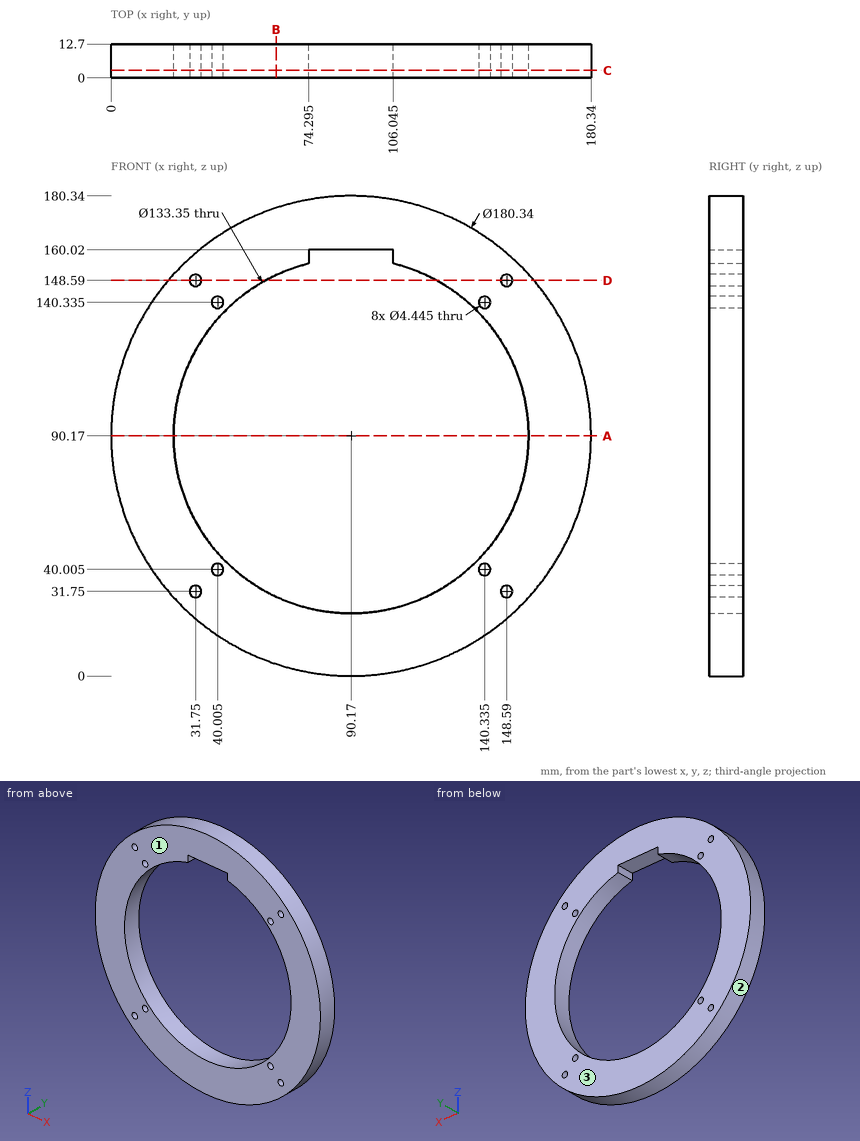
Study the drawing (mm; zero at the part's minimum x, y, z) and answer. Round coordinates to 2 decimals unless told otherwise and drop trailing zeros. Loops run counter-clockwise (first coordinate to the right, second up) from the corner with the lowest first, then second, coordinate; pieces in that order, holes last. Notation, with made-up numbers: (10.5, -1.75) -> (60.5, -1.75) arc R25 cw to (60.5, 10.25) -> close; hole circle Ø10 at (79, 33). An arc over 180 degrees is marked (long way). Write each question's results on one line, items separated by ' | '. Start each with the question number.
1. Section A-A (z = 90.17) is taken. Determine the outline of the cut face in (x, y) (3 decimals), plus the area to 3 significant figures.
2. For a pull along Y with two mould halves and no side action, classify the marked faces 1, 2 and 3 as +Y half, -Y half, draft (parallel to the pull), parting line (faces both ways), or undercut.
3. Section C-C (y = 2.75) is taken. State how many separate pieces and enclosed holes the cut face has, plus the area to 3 significant figures.
4. Section D-D (z = 148.59) is taken. Determine the outline of the cut face in (x, y).
5. Given pin 1 Ø4 at (y, z) = (8, 158) entering from +X; pin 2 Ø4 at (y, z) = (6.5, 158.5) entering from -X; pin 3 Ø1.5 at (x, y) = (119.5, 3.5) entering from -Z, each flat-ended and moving along its own axis, determine where each tip first touches the part or whether it passes through.
6. Find the intervals of material crossed by probe 1 along Z at (x, y) = (85, 9.75); probe 2 along X at (y, z) = (6.25, 148.59); probe 3 along X at (y, z) = (11, 34.5), in increasing order. Write a range as from..to.
7. Section B-B (x = 62) is taken. Determine the outline of the cut face in (y, z), plus the area to 3 significant figures.
Evaluation:
1) outline: (0, 0) -> (23.495, 0) -> (23.495, 12.7) -> (0, 12.7) -> close; (156.845, 0) -> (180.34, 0) -> (180.34, 12.7) -> (156.845, 12.7) -> close | area: 597 mm2
2) face 1: -Y half | face 2: draft | face 3: +Y half
3) separate pieces: 1 | enclosed holes: 9 | area: 11,300 mm2
4) outline: (21.48, 0) -> (29.53, 0) -> (29.53, 12.7) -> (21.48, 12.7) -> close; (33.97, 0) -> (58.03, 0) -> (58.03, 12.7) -> (33.97, 12.7) -> close; (122.31, 0) -> (146.37, 0) -> (146.37, 12.7) -> (122.31, 12.7) -> close; (150.81, 0) -> (158.86, 0) -> (158.86, 12.7) -> (150.81, 12.7) -> close
5) pin 1: stops at x = 151.79 | pin 2: stops at x = 29.09 | pin 3: stops at z = 4.65
6) probe 1: z = 0.15..23.7, 160.02..180.19 | probe 2: x = 21.48..29.53, 33.97..58.03, 122.31..146.37, 150.81..158.86 | probe 3: x = 19.24..53.48, 126.86..161.1
7) outline: (0, 4.51) -> (12.7, 4.51) -> (12.7, 29.74) -> (0, 29.74) -> close; (0, 150.6) -> (12.7, 150.6) -> (12.7, 175.83) -> (0, 175.83) -> close | area: 641 mm2
